CAD build for the part. Positions are in the model's coordinates, mm. A direction names the side the tool comes from. Round coordinates to 2 decimals unless told otherwise and drop trailing zeros. Loops run counter-clockwise (first coordinate to the right, second up) from the corner with the lowest first, then second, coordinate; pieces in that order, holes last. Notation, with made-up numbers: M 40.5,31.5 L 72.5,31.5 A14 ccw 72.5,41.5 Z; hole C -31.75,-6 d4. An arc over 180 degrees is marked long. Use a Markdown table: item, result. Add a question column.
(1) Band-saw the part on C-C, the plane y = -294.5. Write the cut outline in (x, z).
(2) Band-saw the part on A-A, the plane y = -239. Write the cut outline in (x, z) (3 decimals).
(3) Band-saw the part on B-B, the plane z = -58. Write the cut outline in (x, y) (1 decimal), and give its area (3 significant figures).
(4) Two-plate mould, pull along Z, no slides. Class faces 1 (the face through (-93, -228.6, 16)), 2 (the face through (-77.537, -251.618, 81.756)), 3 (the face through (-95, -225.425, -1)): released by +Z, released by -Z, zero draft, split by the parting line, or undercut.
(5) Flat gauge pins, fed straight in: P1, Ø5, axis at x = -86, z = 26.5, coming from the +Y side; P2, Ø4.5, axis at x = -74.5, y = -247, coming from the +Z side; P3, Ø3, axis at x = -75.5, z = -28.5, coming from the +Y side. Where does each tip first touch, or does it go through?
(6) Band-saw the part on D-D, the plane z = -3.5. Write the cut outline in (x, y) (3 decimals).
(7) Which spindle directions (+Z, -Z, +X, -X, +Y, -Y) get a long thin tool onto all of the face, cutting with end or side? Do faces 4 (the face through (-25.4, -265, -1)), 5 (the face through (-93, -247, -25.18)), 6 (the face through (-95, -225.425, -55)), 7 (the face through (-93, -228.6, 68)), 8 (the face through (-93, -228.6, -69)). Say none if no direction does.
(8) Wall check: L1, parallel to Z at x = -104, y = -241; L2, parallel to Z at x = -73, y = -242.5; L3, parallel to Y at x = -68.5, z = 2 (3 decimals). Give the ranges that are in metal, low to high.
from build123d import *

# Parameters (mm, degrees)
REVOLVE1_ANGLE      = 36
SKETCH2_W           = 185.252199215
SKETCH2_H           = 56.371609172
CUT_EXTRUDE1_DEPTH  = 365.059347887
SKETCH5_W           = 55.655123519
SKETCH5_H           = 148.553285118
CUT_EXTRUDE2_DEPTH  = 235.735844279
SKETCH6_W           = 162.024812579
SKETCH6_H           = 19.05
BOSS_EXTRUDE1_DEPTH = 3.175
LPATTERN1_COUNT     = 3
LPATTERN1_PITCH     = 53.34
CUT_EXTRUDE3_DEPTH  = 357.818950588
LPATTERN2_COUNT     = 2
LPATTERN2_PITCH     = 53.34
SKETCH8_W           = 53.705765401
SKETCH8_H           = 196.003453697
CUT_EXTRUDE4_DEPTH  = 224.765760383


with BuildPart() as part:
    # Sketch1 → Revolve1 (revolve, symmetric)
    with BuildSketch(Plane.XY) as revolve1_sk:
        with BuildLine():
            Line((-202.80204389, -227.539822875), (-25.4, -227.539822875))
            Line((-25.4, -227.539822875), (-25.4, -303.739822875))
            ThreePointArc((-25.4, -303.739822875), (-120.294028152, -280.057827584), (-202.80204389, -227.539822875))
        make_face()
    revolve(axis=Axis((0, 0, 0), (-1, 0, 0)), revolution_arc=REVOLVE1_ANGLE / 2)
    revolve(revolve1_sk.sketch, axis=Axis((0, 0, 0), (1, 0, 0)), revolution_arc=REVOLVE1_ANGLE / 2)

    # Sketch2 → Cut-Extrude1 (cut, through all)
    with BuildSketch(Plane(origin=(-25.4, 0, 0), x_dir=(0, 0, -1), z_dir=(1, 0, 0))):
        with Locations((3.182919918, -200.414195414)):
            Rectangle(SKETCH2_W, SKETCH2_H)
    extrude(amount=-CUT_EXTRUDE1_DEPTH, mode=Mode.SUBTRACT)

    # Sketch5 → Cut-Extrude2 (cut, through all)
    with BuildSketch(Plane(origin=(0, -228.6, 0), x_dir=(1, 0, 0), z_dir=(0, 1, 0))):
        with Locations((-215.252374339, 0)):
            Rectangle(SKETCH5_W, SKETCH5_H)
    extrude(amount=-CUT_EXTRUDE2_DEPTH, mode=Mode.SUBTRACT)

    # Sketch6 → Boss-Extrude1 (add)
    with BuildSketch(Plane(origin=(0, -228.6, 0), x_dir=(1, 0, 0), z_dir=(0, 1, 0))):
        with Locations((-106.41240629, -52.051642559)):
            Rectangle(SKETCH6_W, SKETCH6_H)
    boss_extrude1 = extrude(amount=BOSS_EXTRUDE1_DEPTH)

    # LPattern1: Boss-Extrude1 ×3
    with Locations(*[(0, 0, -i * LPATTERN1_PITCH) for i in range(1, LPATTERN1_COUNT)]):
        add(boss_extrude1)

    # Sketch7 → Cut-Extrude3 (cut, through all)
    with BuildSketch(Plane(origin=(-25.4, 0, 0), x_dir=(0, 0, -1), z_dir=(1, 0, 0))):
        with BuildLine():
            Line((-22.603517559, -244.856), (-22.603517559, -248.92))
            Line((-22.603517559, -248.92), (-28.159767559, -248.92))
            Line((-28.159767559, -248.92), (-28.159767559, -244.856))
            Line((-28.159767559, -244.856), (-30.144142559, -244.856))
            Line((-30.144142559, -244.856), (-30.144142559, -241.427))
            ThreePointArc((-30.144142559, -241.427), (-30.23394512, -241.210197439), (-30.017142559, -241.3))
            Line((-30.017142559, -241.3), (-28.159767559, -241.3))
            Line((-28.159767559, -241.3), (-28.159767559, -228.6))
            Line((-28.159767559, -228.6), (-22.603517559, -228.6))
            Line((-22.603517559, -228.6), (-22.603517559, -241.3))
            Line((-22.603517559, -241.3), (-20.746142559, -241.3))
            ThreePointArc((-20.746142559, -241.3), (-20.529339998, -241.210197439), (-20.619142559, -241.427))
            Line((-20.619142559, -241.427), (-20.619142559, -244.856))
            Line((-20.619142559, -244.856), (-22.603517559, -244.856))
        make_face()
    cut_extrude3 = extrude(amount=-CUT_EXTRUDE3_DEPTH, mode=Mode.SUBTRACT)

    # LPattern2: Cut-Extrude3 ×2
    with Locations(*[(0, 0, -i * LPATTERN2_PITCH) for i in range(1, LPATTERN2_COUNT)]):
        add(cut_extrude3, mode=Mode.SUBTRACT)

    # Sketch8 → Cut-Extrude4 (cut, through all)
    with BuildSketch(Plane(origin=(0, -225.425, 0), x_dir=(1, 0, 0), z_dir=(0, 1, 0))):
        with Locations((-188.777882701, -12.617417505)):
            Rectangle(SKETCH8_W, SKETCH8_H)
    extrude(amount=-CUT_EXTRUDE4_DEPTH, mode=Mode.SUBTRACT)


solid = part.part
Return value:
| question | item | result |
|---|---|---|
| 1 | outline | M -25.4,-74.35 L -25.4,74.35 A78.57 ccw Z |
| 2 | outline | M -161.925,-77.656 L -25.4,-77.656 L -25.4,-30.736 L -161.925,-30.736 Z; M -161.925,-25.18 L -25.4,-25.18 L -25.4,22.604 L -161.925,22.604 Z; M -161.925,28.16 L -25.4,28.16 L -25.4,77.656 L -161.925,77.656 Z |
| 3 | outline | M -161.9,-251.6 A299.2 ccw -25.4,-298.2 L -25.4,-225.4 L -161.9,-225.4 Z |
| 3 | area | 7,600 mm^2 |
| 4 | face 1 | undercut |
| 4 | face 2 | released by +Z |
| 4 | face 3 | zero draft |
| 5 | P1 | y = -228.6 |
| 5 | P2 | z = 80.99 |
| 5 | P3 | y = -248.92 |
| 6 | outline | M -161.925,-258.207 A304.78 ccw -25.4,-303.72 L -25.4,-225.425 L -161.925,-225.425 Z |
| 7 | face 4 | +Z, -Z, +X, +Y, -Y |
| 7 | face 5 | +X, -X, +Y |
| 7 | face 6 | +Z, -Z, +X, -X, +Y |
| 7 | face 7 | +Z, +X, -X, +Y |
| 7 | face 8 | -Z, +X, -X, +Y |
| 8 | L1 | -78.31 to -30.74, -25.18 to 22.6, 28.16 to 78.31 |
| 8 | L2 | -78.79 to -32.72, -23.2 to 20.62, 30.14 to 78.79 |
| 8 | L3 | -296.996 to -225.425 |
